Autodesk Inventor part; units mm, degrees
sketch "Sketch5" plane through (0, 0, 0) normal (1, 0, 0) x (0, 1, 0)
  line L0 (-8.5, 10) -> (0, 10)
  line L1 (0, 10) -> (0, -10)
  line L2 (0, -10) -> (-14.4, -10)
  line L3 (-15.4, -9) -> (-15.4, 10)
  line L4 (-26.0485, 0) -> (4.3414, 0)
  line L5 (0, -16.9345) -> (0, 30.1575)
  line L6 (-14.5, 23.223) -> (-20.5, 23.223)
  line L7 (-21.5, 22.223) -> (-21.5, 17)
  ellipse E0 centre (-21.5, 10) end of major axis (-21.5, 17) minor radius 6.1 (-15.4, 10) -> (-21.5, 17) ccw
  line L8 (-13.5, 22.223) -> (-13.5, 15)
  arc A0 (-20.5, 23.223) -> (-21.5, 22.223) centre (-20.5, 22.223) ccw
  arc A1 (-13.5, 22.223) -> (-14.5, 23.223) centre (-14.5, 22.223) ccw
  arc A2 (-15.4, -9) -> (-14.4, -10) centre (-14.4, -9) ccw
  arc A3 (-13.5, 15) -> (-8.5, 10) centre (-8.5, 15) ccw
  point P0 (0, 0)
  point P1 (-15.4, -10)
  point P2 (-13.5, 10)
  dimension "d64" = 6.1
  dimension "d78" = 7
  dimension "d31" = 15.4
  dimension "d32" = 20
  dimension "d33" = 10
  dimension "d34" = 15.4
  dimension "d58" = 21.5
  dimension "d59" = 23.223
  dimension "d71" = 8
  dimension "d74" = 1
  dimension "d75" = 1
  dimension "d76" = 0
  dimension "d77" = 5
extrude "Extrusion4" add sketch "Sketch5" along normal mid plane 7.4
sketch "Sketch6" plane through (-3.7, -15.4, -10) normal (0, -1, 0) x (1, 0, 0)
  circle A0 centre (3.7, 10) radius 2
  line L0 (3.7, 39.8676) -> (3.7, -6.6446)
  point P0 (3.7, 10)
  dimension "d37" = 4
extrude "Extrusion5" cut sketch "Sketch6" against normal blind 15.5
sketch "Sketch7" plane through (-3.7, 0, 0) normal (-1, 0, 0) x (0, 0, 1)
  circle A0 centre (0, -7.4) radius 7
  line L0 (10, 0) -> (-10, 0)
  line L1 (0, -25.8) -> (0, 4.3)
  circle A1 centre (0, -7.4) radius 4
  point P0 (0, 0)
  dimension "d40" = 14
  dimension "d41" = 7.4
  dimension "d42" = 0
  dimension "d43" = 8
extrude "Extrusion6" add sketch "Sketch7" along normal blind 16.2 contours A0 L1 A1 | L1 A1 A0
sketch "Sketch8" plane through (-19.9, -7.4, 0) normal (-1, 0, 0) x (0, 0, 1)
  circle A0 centre (0, 0) radius 6.5
  line L0 (0, 11.7) -> (0, -18.4)
  line L1 (10, 7.4) -> (-10, 7.4)
  point P0 (0, 7.4)
  dimension "d46" = 13
  dimension "d47" = 0
  dimension "d48" = 7.4
extrude "Extrusion7" cut sketch "Sketch8" against normal blind 12.3
sketch "Sketch10" plane through (-3.7, -21.5, 17) normal (0, -1, 0) x (1, 0, 0)
  circle A0 centre (3.7, 2.223) radius 1.5
  line L0 (-1.48, -17) -> (8.88, -17)
  line L1 (3.7, 12.8676) -> (3.7, -33.6446)
  point P0 (3.7, -17)
  dimension "d82" = 3
  dimension "d83" = 19.223
  dimension "d84" = 0
extrude "Extrusion8" cut sketch "Sketch10" against normal blind 8
fillet "Fillet1" radius 1 1 edges at (0, 0, -10)
fillet "Fillet2" radius 1 1 edges at (0, 0, 10)
properties part number "support_avant"
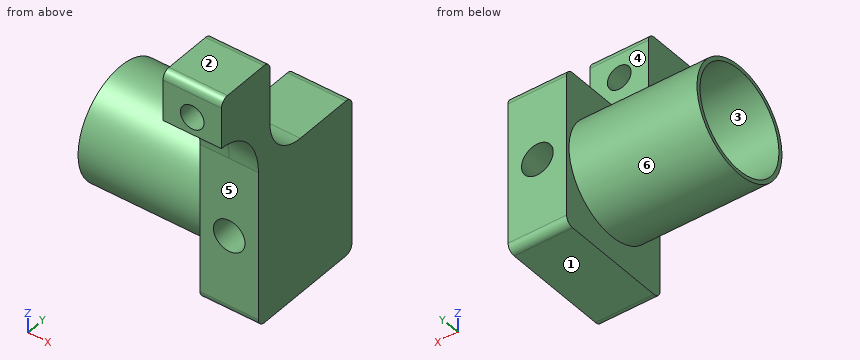
For this review, take the finished solid that the model builds, in its own axes (mm). Face numbers are marked on the shaded views. A direction names the side the tool comes from. Coordinates: 2 decimals unless noted, no trailing zeros. Loops run counter-clockwise (first coordinate to the right, second up) from the corner with the lowest first, then second, coordinate; pieces in that order, holes last. Notation, with made-up numbers: (40.25, 58) - (86.25, 58) arc R18 ccw to (86.25, 91) - close; hole circle Ø2 at (-26.5, 31.25). An arc over 180 degrees is marked (long way). Use a Markdown table: item, result. Add a question column.
Item 1: Tool access review of the marked faces 4, 5 and 6: name each direction out of +Z, -Z, +X, -X, +Y, -Y from which nothing blocks a thin tool from reaching the whole face with its end or side.
Item 2: Mouldability with a two-part tool opening along Z and no side actions: class the marked faces 1, 2 and 3 as pulls with the +Z half, pulls with the -Z half, needs draft (parallel to the pull), parting line crosses it, or undercut.
Item 3: We need section A-A (y = -7.4). Give the boundary of the cut face in (x, z), and give its area (3 significant figures).
Item 4: We need section D-D (y = -10). Give the boundary of the cut face in (x, z), and give its area (3 significant figures).
Item 5: We need section C-C (x = -14.25). Give the boundary of the cut face in (y, z), and give its area (3 significant figures).
Item 6: Insertion check: pin 1 Ø1 at (y, z) = (-11.5, 7.5) entering from -X; pin 2 Ø3.5 at (x, z) = (0, 19.223) entering from +Y; pin 3 Ø4 at (x, z) = (-3, -2.5) entering from -Y; pin 4 Ø3 at (x, z) = (0, 0) entering from -Y. Each pin has a flat end and moves straight along its axis. Give the tip position at first contact, or say it passes through.
Item 7: We need section B-B (z = 0). Give the boundary of the cut face in (x, y), and give its area (3 significant figures).
Item 8: For line 1 (Z direction, x = -5.85, y = -7.4); line 2 (Y direction, x = -6.2, z = 0); line 3 (Z direction, x = -17.75, y = -7.5), list the stretches that pass through material, from the lowest coordinate up.
Results list:
| question | item | result |
|---|---|---|
| 1 | face 4 | +Z, +X, -X, +Y |
| 1 | face 5 | -Z, +X, -X, -Y |
| 1 | face 6 | -X |
| 2 | face 1 | pulls with the -Z half |
| 2 | face 2 | pulls with the +Z half |
| 2 | face 3 | undercut |
| 3 | outline | (-19.9, -7) - (-3.7, -7) - (-3.7, -10) - (3.7, -10) - (3.7, 10) - (-3.7, 10) - (-3.7, 7) - (-19.9, 7) - (-19.9, 6.5) - (-7.6, 6.5) - (-7.6, 4) - (-3.7, 4) - (-3.7, -4) - (-7.6, -4) - (-7.6, -6.5) - (-19.9, -6.5) - close; hole circle Ø4 at (0, 0) |
| 3 | area | 171 mm^2 |
| 4 | outline | (-19.9, -6.5) - (-3.7, -6.5) - (-3.7, -10) - (3.7, -10) - (3.7, 10.23) - (-3.7, 10.23) - (-3.7, 6.5) - (-19.9, 6.5) - (-19.9, 5.96) - (-7.6, 5.96) - (-7.6, 3.04) - (-3.7, 3.04) - (-3.7, -3.04) - (-7.6, -3.04) - (-7.6, -5.96) - (-19.9, -5.96) - close; hole circle Ø4 at (0, 0) |
| 4 | area | 177 mm^2 |
| 5 | outline | circle Ø14 at (-7.4, 0); hole circle Ø13 at (-7.4, 0) |
| 5 | area | 21.2 mm^2 |
| 6 | pin 1 | stops at x = -3.7 |
| 6 | pin 2 | stops at y = -13.5 |
| 6 | pin 3 | stops at y = -15.4 |
| 6 | pin 4 | passes through |
| 7 | outline | (-19.9, -14.4) - (-3.7, -14.4) - (-3.7, -15.4) - (-2, -15.4) - (-2, 0) - (-3.7, 0) - (-3.7, -0.4) - (-19.9, -0.4) - (-19.9, -0.9) - (-7.6, -0.9) - (-7.6, -3.4) - (-3.7, -3.4) - (-3.7, -11.4) - (-7.6, -11.4) - (-7.6, -13.9) - (-19.9, -13.9) - close; (2, -15.4) - (3.7, -15.4) - (3.7, 0) - (2, 0) - close |
| 7 | area | 88.1 mm^2 |
| 8 | line 1 | z = -7 to -4, 4 to 7 |
| 8 | line 2 | y = -14.4 to -11.4, -3.4 to -0.4 |
| 8 | line 3 | z = -7 to -6.5, 6.5 to 7 |
